Geometry: final body of the model. Coordinates: model frame, mm. A direction names the side the tool comes from. Give positions to 0.01 mm unless a question says otherwise; leave off trailing zeros. Write each loop counter-clockwise with the first axis right and the second up, starting at its lowest first coordinate (ties: lowest second). Pieces come first, ordered by that corner, then holes. Notation, with made-up numbers: M -4,4 L 13,4 A23 cw 13,20 Z; hole C 61,-13.5 d10. An arc over 180 degrees is marked long. Use a Markdown table: item, result. Add a question column.
(1) Draft query along Z for faces 1 (the cylindrical face through (37.56, 177.06, 23.95)), 2 (the cylindrical face through (39.702, 177.064, 25.312)), 3 (the flat face through (-35, 0, -28)). Return one class per face: released by +Z, released by -Z, zero draft, split by the parting line, or undercut.
(2) Cut plane C-C (z = 23). Output: boundary loops of the cut face in (x, y), plus the area to 3 significant figures.
(3) Cut plane A-A (x = 0). Output: boundary loops of the cut face in (y, z), plus the area to 3 significant figures.
(4) Cut plane D-D (y = 252.5). Output: boundary loops of the cut face in (x, z), plus the area to 3 significant figures.
(5) Material intervals for L1, parallel to X at y = 185, z = 0; L2, parallel to Z at x = -2, y = 335; L3, parallel to Z at x = -24.5, y = 119, sorted ascending.
(6) Pin query (flat end, axial travel): pin 1 Ø4 at (x, y) = (28.5, 40) entering from -Z; pin 2 Ø2 at (x, y) = (-42.5, 276.5) entering from +Z; pin 3 Ø12 at (x, z) = (35.5, 31) entering from +Y; pin 4 Ø1 at (x, y) = (24.5, 59.5) entering from -Z. Return the tip coordinate at first contact, or that it passes through.
(7) Reachability of faces 4 (the flat face through (-35, 359.156, -28)), 5 (the flat face through (-45, 302.695, -2)) from +Z, -Z, +X, -X, +Y, -Y: full face, straight path, thin tool, end or side. Return the list, or none.
(8) Cut plane B-B (z = 0). Output: boundary loops of the cut face in (x, y), plus the area to 3 significant figures.
```python
from build123d import *

# Parameters (mm, degrees)
SKETCH1_R           = 47.084225238
BOSS_EXTRUDE1_DEPTH = 359.156
SHELL1_T            = -2.54
SKETCH2_W           = 31.043805041
SKETCH2_H           = 64.909774176
CUT_EXTRUDE1_DEPTH  = 359.156


with BuildPart() as part:
    # Sketch1 → Boss-Extrude1 (new body)
    with BuildSketch(Plane(origin=(0, 0, 0), x_dir=(1, 0, 0), z_dir=(0, 1, 0))):
        with Locations(Location((0, 0, 0), (0, 0, 270))):
            Circle(SKETCH1_R)
    extrude(amount=BOSS_EXTRUDE1_DEPTH)

    # Shell1
    shell1_openings = [part.faces().sort_by_distance(p)[0] for p in [
        (0, 359.156, 0),
        (0, 0, 0),
    ]]
    offset(amount=SHELL1_T, openings=shell1_openings, kind=Kind.INTERSECTION)

    # Sketch2 → Cut-Extrude1 (cut)
    with BuildSketch(Plane(origin=(0, 0, 0), x_dir=(0, 0, -1), z_dir=(1, 0, 0))):
        with Locations((2.351803412, 270.240021539)):
            Rectangle(SKETCH2_W, SKETCH2_H)
    extrude(amount=-CUT_EXTRUDE1_DEPTH, mode=Mode.SUBTRACT)


solid = part.part
```
Answer list:
| question | item | result |
|---|---|---|
| 1 | face 1 | undercut |
| 1 | face 2 | split by the parting line |
| 1 | face 3 | zero draft |
| 2 | outline | M -41.08,0 L -38.15,0 L -38.15,359.16 L -41.08,359.16 Z; M 38.15,0 L 41.08,0 L 41.08,359.16 L 38.15,359.16 Z |
| 2 | area | 2,110 mm² |
| 3 | outline | M 0,-47.08 L 359.16,-47.08 L 359.16,-44.54 L 0,-44.54 Z; M 0,44.54 L 359.16,44.54 L 359.16,47.08 L 0,47.08 Z |
| 3 | area | 1,820 mm² |
| 4 | outline | M -45.2,13.17 L -42.55,13.17 A44.54 cw long -40.8,-17.87 L -43.56,-17.87 A47.08 ccw long Z |
| 4 | area | 651 mm² |
| 5 | L1 | -47.08 to -44.54, 44.54 to 47.08 |
| 5 | L2 | -47.04 to -44.5, 44.5 to 47.04 |
| 5 | L3 | -40.21 to -37.2, 37.2 to 40.21 |
| 6 | pin 1 | z = -38.92 |
| 6 | pin 2 | z = 22.24 |
| 6 | pin 3 | y = 359.16 |
| 6 | pin 4 | z = -40.51 |
| 7 | face 4 | +Z, -Z, +X, -X, +Y |
| 7 | face 5 | -X |
| 8 | outline | M -47.08,0 L -44.54,0 L -44.54,237.79 L -47.08,237.79 Z; M -47.08,302.69 L -44.54,302.69 L -44.54,359.16 L -47.08,359.16 Z; M 44.54,0 L 47.08,0 L 47.08,359.16 L 44.54,359.16 Z |
| 8 | area | 1,660 mm² |
